Check sheet for the drawn part. Datum: minimum x, y, z corner. Units: mm. A direction names the side the tool comes from. Round coordinates to 2 decimals unless told otherwise and drop trailing zeros. Order: outer loops, then holes, each group sorted by start corner. A loop starts at its lowest first (then second) coordinate and runs counter-clockwise, first axis right, second up. Notation, with made-up numbers: (-3, 59.5) - (50, 59.5) arc R27 cw to (50, 87.5) - close; hole circle Ø1 at (59.5, 80). An arc over 180 degrees is marked (long way). Write each question's results on one line, items separated by ' | '.
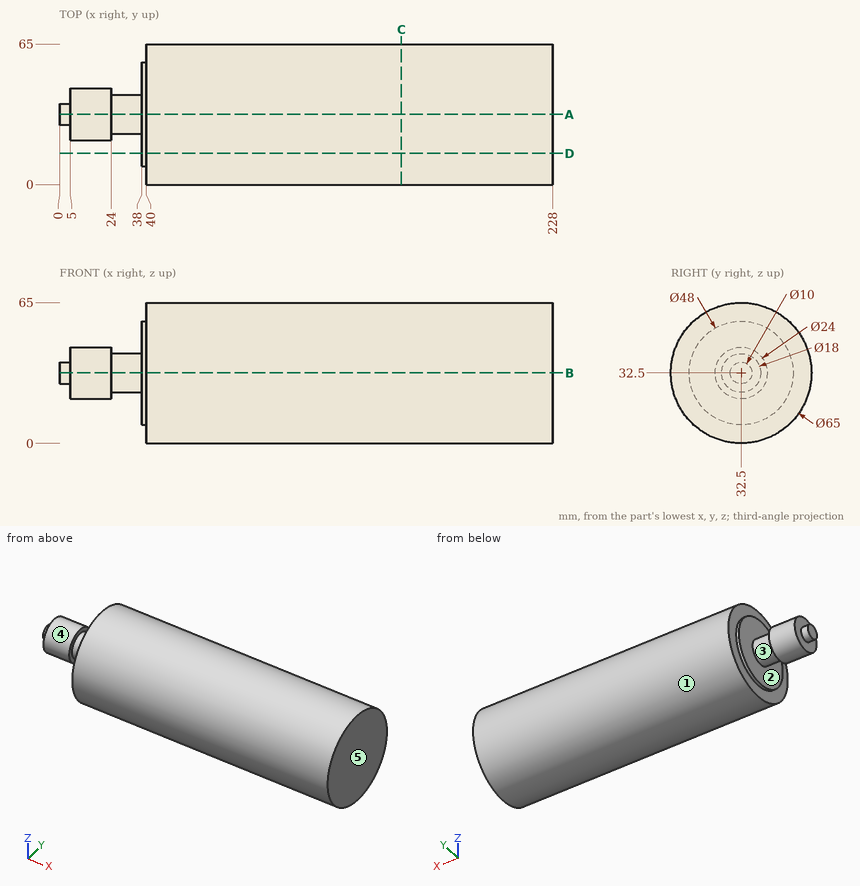
(1) Section check D-D (y = 14.5). Record the cut outline in (x, z), then the cut area to 3 significant figures.
Answers follow:
outline: (38, 16.63) - (40, 16.63) - (40, 5.44) - (228, 5.44) - (228, 59.56) - (40, 59.56) - (40, 48.37) - (38, 48.37) - close | area: 10,200 mm²
(2) Draft check along X on the marked faces 3, 4 and 5. Enter one of: released by +X, released by -X, zero draft, split by the parting line, or undercut.
Answers follow:
face 3: undercut | face 4: zero draft | face 5: released by +X
(3) Material ranges on line 1 (X direction, y = 12, z = 46); line 2 (Z direction, x = 128, y = 34); line 3 (X direction, y = 10.5, z = 28), recorded low to high.
Answers follow:
line 1: 40 to 228 | line 2: 0.03 to 64.97 | line 3: 38 to 228
(4) Section check C-C (x = 158). Record the cut outline in (y, z).
Answers follow:
outline: circle Ø65 at (32.5, 32.5)
(5) Depth check by flat-ended pin: pin 1 Ø1 at (x, y) = (120.5, 43) entering from -Z; pin 2 Ø8 at (x, y) = (181.5, 35) entering from +Z; pin 3 Ø4 at (y, z) = (38.5, 18) entering from -X. Enter the tip coordinate at first touch or a pass-through.
Answers follow:
pin 1: z = 1.58 | pin 2: z = 65 | pin 3: x = 38
(6) Section check A-A (y = 32.5). Record the cut outline in (x, z), then the cut area to 3 significant figures.
Answers follow:
outline: (0, 27.5) - (5, 27.5) - (5, 20.5) - (24, 20.5) - (24, 23.5) - (38, 23.5) - (38, 8.5) - (40, 8.5) - (40, 0) - (228, 0) - (228, 65) - (40, 65) - (40, 56.5) - (38, 56.5) - (38, 41.5) - (24, 41.5) - (24, 44.5) - (5, 44.5) - (5, 37.5) - (0, 37.5) - close | area: 13,100 mm²
(7) Access from +Z, -Z, +X, -X, +Y, -Y to the whole of each face (thin tool, end or side, straight path). Record for the marked faces 1 and 2.
Answers follow:
face 1: +X, -X | face 2: none
